from build123d import *

# Parameters (mm, degrees)
SKETCH1_R          = 13.890625
SKETCH1_R_2        = 8.89
SKETCH3_R          = 10.7696
CUT_EXTRUDE1_DEPTH = 19.05
SKETCH4_R          = 10.7696
CUT_EXTRUDE2_DEPTH = 19.05


with BuildPart() as part:
    # Sweep1: sweep along a path in Sketch2
    with BuildLine(Plane(origin=(0, 0, 0), x_dir=(0, 0, -1), z_dir=(1, 0, 0))) as sweep1_path:
        Line((0, 0), (17.78, 0))
        ThreePointArc((17.78, 0), (27.658281733, 4.091718267), (31.75, 13.97))
        Line((31.75, 13.97), (31.75, 31.75))
    # Sketch1 → Sweep1 (sweep)
    with BuildSketch(Plane.XY):
        Circle(SKETCH1_R)
        Circle(SKETCH1_R_2, mode=Mode.SUBTRACT)
    sweep(path=sweep1_path.line)

    # Sketch3 → Cut-Extrude1 (cut)
    with BuildSketch(Plane.XY):
        Circle(SKETCH3_R)
    extrude(amount=-CUT_EXTRUDE1_DEPTH, mode=Mode.SUBTRACT)

    # Sketch4 → Cut-Extrude2 (cut)
    with BuildSketch(Plane(origin=(0, 31.75, 0), x_dir=(1, 0, 0), z_dir=(0, 1, 0))):
        with Locations((0, 31.75)):
            Circle(SKETCH4_R)
    extrude(amount=-CUT_EXTRUDE2_DEPTH, mode=Mode.SUBTRACT)


solid = part.part
Can you work these out from the model? Positions are in its coordinate system, mm. A direction names the side the tool comes from. Round coordinates to 2 decimals unless told otherwise and drop trailing zeros. Order: outer loops, then holes, each group sorted by start corner. A loop starts at its lowest first (then second) coordinate and runs counter-clockwise, first axis right, second up. Notation, with made-up numbers: (75, -14.5) - (119, -14.5) arc R29 cw to (119, 10.5) - close; hole circle Ø4 at (-11.75, 5). An arc over 180 degrees is marked (long way). Answer in a Markdown table with one row per item.
(1) Suppose I cut it at B-B, the plane y = 20.5. Please give me the cut outline in (x, z).
From the geometry:
| item | result |
|---|---|
| outline | circle Ø27.78 at (0, -31.75); hole circle Ø21.54 at (0, -31.75) |
(2) Which directions (+Z, -Z, +X, -X, +Y, -Y) give clear straight access to the entire face, cutting with the end or side of a thin tool? Please do faces 1 (the face through (-10.2, 31.75, -35.8)), 2 (the face through (-2, 9, -19.05)), 3 (the face through (-3.01, 22.98, -18.19)).
From the geometry:
| item | result |
|---|---|
| face 1 | +Z, -Z, +X, -X, +Y |
| face 2 | +Z |
| face 3 | +Y |
(3) For P1, Ø1.5, axis at x = 1, y = 13.5, coming from the -Z side; P2, Ø10, axis at x = 2.5, y = 26.5, coming from the +Z side; P3, Ø6.5, axis at x = 3, z = -37, coming from the +Y side, each with a flat end and sliding along its axis, tell me the tip position at first contact or that it passes through.
From the geometry:
| item | result |
|---|---|
| P1 | stops at z = -45.64 |
| P2 | stops at z = -17.86 |
| P3 | stops at y = 12.7 |
(4) Please list where these lines run through material, in increasing order: L1, parallel to Z at x = 0, y = 17.5; L2, parallel to X at y = 18, z = -31.75; L3, parallel to X at y = -3, z = -21.5. Write a range as from..to.
From the geometry:
| item | result |
|---|---|
| L1 | z = -45.64..-42.52, -20.98..-17.86 |
| L2 | x = -13.89..-10.77, 10.77..13.89 |
| L3 | x = -13.47..-8.21, 8.21..13.47 |
(5) Suppose I cut it at A-A, the plane x = 1.5. Please give me the cut outline in (y, z).
From the geometry:
| item | result |
|---|---|
| outline | (-13.81, -17.78) arc R27.78 ccw to (13.97, -45.56) - (31.75, -45.56) - (31.75, -42.41) - (12.7, -42.41) - (12.7, -40.48) arc R22.73 cw to (-8.73, -19.05) - (-10.66, -19.05) - (-10.66, 0) - (-13.81, 0) - close; (8.92, -19.05) arc R5.21 ccw to (12.7, -22.83) - (12.7, -21.09) - (31.75, -21.09) - (31.75, -17.94) - (13.97, -17.94) arc R0.16 cw to (13.81, -17.78) - (13.81, 0) - (10.66, 0) - (10.66, -19.05) - close |
(6) If we mould it in two halves opening along X, with no side actions, what happens to faces 4 (the face through (4.1, -10.2, 0)), 5 (the face through (-1.808, -13.772, -9.014)), 6 (the face through (-1, 12.7, -41))? For each: released by +X, released by -X, zero draft, split by the parting line, or undercut.
From the geometry:
| item | result |
|---|---|
| face 4 | zero draft |
| face 5 | split by the parting line |
| face 6 | undercut |
(7) Suppose I cut it at D-D, the plane x = -4.5. Please give me the cut outline in (y, z).
From the geometry:
| item | result |
|---|---|
| outline | (-13.14, -17.78) arc R27.11 ccw to (13.97, -44.89) - (31.75, -44.89) - (31.75, -41.53) - (12.7, -41.53) - (12.7, -39.38) arc R21.64 cw to (-7.63, -19.05) - (-9.78, -19.05) - (-9.78, 0) - (-13.14, 0) - close; (7.8, -19.05) arc R6.3 ccw to (12.7, -23.95) - (12.7, -21.97) - (31.75, -21.97) - (31.75, -18.61) - (13.97, -18.61) arc R0.83 cw to (13.14, -17.78) - (13.14, 0) - (9.78, 0) - (9.78, -19.05) - close |
(8) Suppose I cut it at C-C, the plane z = -6.5. Please give me the cut outline in (x, y).
From the geometry:
| item | result |
|---|---|
| outline | circle Ø27.78 at (0, 0); hole circle Ø21.54 at (0, 0) |
